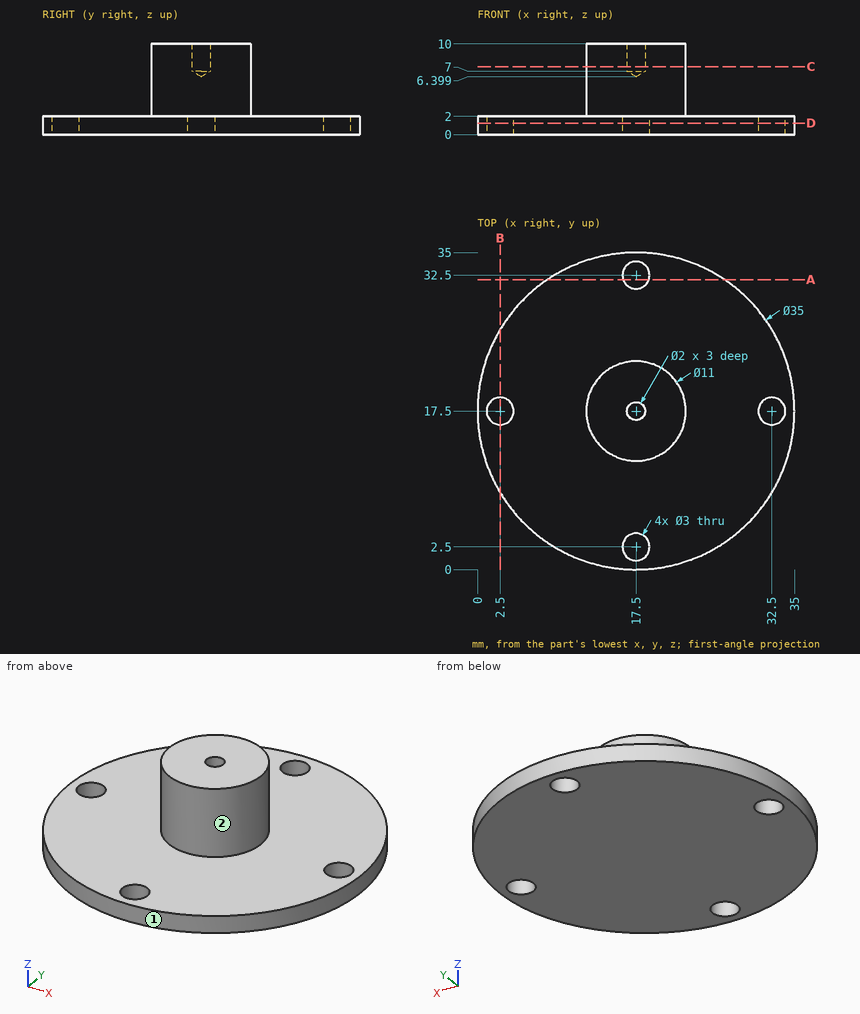
Study the drawing (mm; zero at the part's minimum x, y, z) and answer. A direction names the side the tool comes from. Give positions to 0.01 mm unless a question says otherwise; leave off trailing zeros. Loops run counter-clockwise (first coordinate to the right, second up) from the corner with the lowest first, then second, coordinate; pieces in that order, holes last. Notation, with made-up numbers: (61, 84.5) - (103, 84.5) arc R23 ccw to (103, 101.5) - close; hole circle Ø10 at (23.5, 5.5). An arc over 180 degrees is marked (long way). Answer in a Markdown table with one row per item. Add a question column.
Q1. A tool of negligible diameter and unlimited length cuts with its end or side. For the marked faces 1 and 2, from which of +Z, -Z, +X, -X, +Y, -Y can it reach the whole face along a straight path? Write none if from no direction.
Q2. The part is cut by section B-B (x = 2.5). Determine the outline of the cut face in (y, z).
Q3. The part is cut by section C-C (z = 7.5). Determine the outline of the cut face in (x, y), and give its area (3 significant figures).
Q4. Consider line 1 along Y through (x, z) = (17.5, 1.15); line 2 along Y through (x, z) = (17.5, 8.2); line 3 along Y through (x, z) = (18, 1). Determine where each line is inside the solid, lowest interval first.
Q5. The part is cut by section A-A (y = 32). Determine the outline of the cut face in (x, z).
Q6. The part is cut by section D-D (z = 1.25). Determine the outline of the cut face in (x, y).
Q7. Each of these flat-tipped pins is pushed along its axis until it touches: P1, Ø2, axis at x = 31, y = 28, coming from the +Z side; P2, Ø2.5, axis at x = 17.5, y = 17.5, coming from the +Z side; P3, Ø1.5, axis at x = 20.5, z = 5, coming from the +Y side. Where does it stop, or does it pass through?
Solution:
| question | item | result |
|---|---|---|
| 1 | face 1 | +Z, -Z |
| 1 | face 2 | +Z |
| 2 | outline | (8.49, 0) - (16, 0) - (16, 2) - (8.49, 2) - close; (19, 0) - (26.51, 0) - (26.51, 2) - (19, 2) - close |
| 3 | outline | circle Ø11 at (17.5, 17.5); hole circle Ø2 at (17.5, 17.5) |
| 3 | area | 91.9 mm² |
| 4 | line 1 | y = 0 to 1, 4 to 31, 34 to 35 |
| 4 | line 2 | y = 12 to 16.5, 18.5 to 23 |
| 4 | line 3 | y = 0.01 to 1.09, 3.91 to 31.09, 33.91 to 34.99 |
| 5 | outline | (7.7, 0) - (16.09, 0) - (16.09, 2) - (7.7, 2) - close; (18.91, 0) - (27.3, 0) - (27.3, 2) - (18.91, 2) - close |
| 6 | outline | circle Ø35 at (17.5, 17.5); hole circle Ø3 at (2.5, 17.5); hole circle Ø3 at (17.5, 2.5); hole circle Ø3 at (17.5, 32.5); hole circle Ø3 at (32.5, 17.5) |
| 7 | P1 | stops at z = 2 |
| 7 | P2 | stops at z = 10 |
| 7 | P3 | stops at y = 22.52 |
